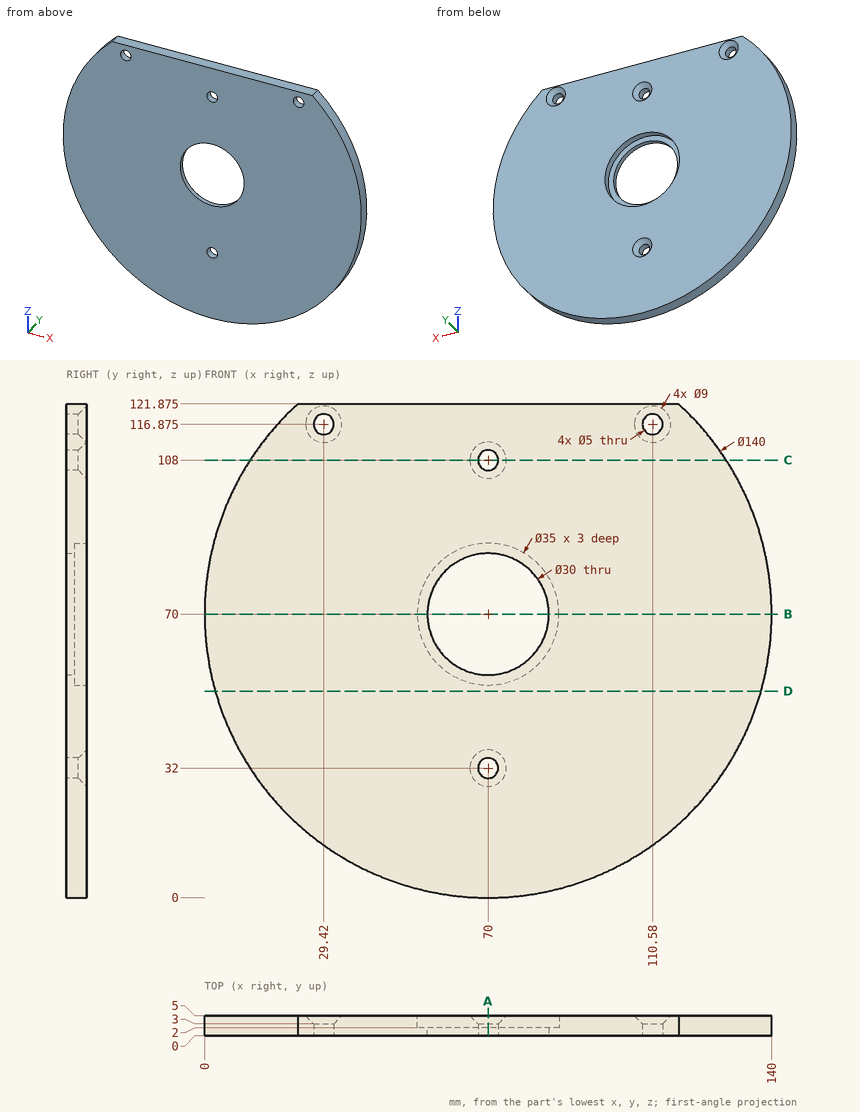
Geometry check sheet. Reference: drawing and pictorial views, mm from the part's lowest x, y, z. Round coordinates to 2 decimals unless told otherwise and drop trailing zeros. Write each loop counter-clockwise with the first axis right and the second up, starting at its lowest first coordinate (ties: lowest second). Pieces come first, ordered by that corner, then holes. Notation, with made-up numbers: (-12, -20) -> (10, -20) arc R19 ccw to (10, -6) -> close; hole circle Ø7 at (-25, 54). An arc over 180 degrees is marked (long way). Put each result on its own line as item: value.
1) Depth check by flat-ended pin: P1, Ø3, axis at y = 3.5, z = 49, coming from the -X side; P2, Ø6, axis at x = 29.42, z = 116.87, coming from the +Y side (1 decimal); P3, Ø3, axis at x = 70, z = 108, coming from the +Y side; P4, Ø6.5, axis at x = 70, z = 32, coming from the +Y side. Enter the tip coordinate at first touch or a pass-through.
Recorded:
P1: stops at x = 2.77
P2: stops at y = 3.5
P3: passes through
P4: stops at y = 3.75
2) Thickness scan on probe 1 along Z at (x, y) = (70, 0.8) (3 decimals); probe 2 along Z at (x, y) = (86.5, 0.7) (1 decimal); probe 3 along X at (y, z) = (0.3, 81.5). Record the ranges inside material, lowest first. Write a range as from..to.
Recorded:
probe 1: z = 0..29.5, 34.5..55, 85..105.5, 110.5..121.875
probe 2: z = 2..121.9
probe 3: x = 0.95..60.37, 79.63..139.05
3) Cross-section at C-C, the plane z = 108. Enter the section's corners in (x, y), plus the area to 3 significant figures.
Recorded:
outline: (11.21, 0) -> (67.5, 0) -> (67.5, 3) -> (65.5, 5) -> (11.21, 5) -> close; (72.5, 0) -> (128.79, 0) -> (128.79, 5) -> (74.5, 5) -> (72.5, 3) -> close
area: 559 mm2
4) Cross-section at D-D, the plane z = 51. Enter the section's corners in (x, y), plus the area to 3 significant figures.
Recorded:
outline: (2.63, 0) -> (137.37, 0) -> (137.37, 5) -> (2.63, 5) -> close
area: 674 mm2
5) Cross-section at B-B, the plane z = 70. Enter the section's corners in (x, y).
Recorded:
outline: (0, 0) -> (55, 0) -> (55, 2) -> (52.5, 2) -> (52.5, 5) -> (0, 5) -> close; (85, 0) -> (140, 0) -> (140, 5) -> (87.5, 5) -> (87.5, 2) -> (85, 2) -> close
6) Cross-section at A-A, the plane x = 70. Enter the section's corners in (y, z) (3 decimals), plus the area to 3 significant figures.
Recorded:
outline: (0, 0) -> (5, 0) -> (5, 27.5) -> (3, 29.5) -> (0, 29.5) -> close; (0, 34.5) -> (3, 34.5) -> (5, 36.5) -> (5, 52.5) -> (2, 52.5) -> (2, 55) -> (0, 55) -> close; (0, 85) -> (2, 85) -> (2, 87.5) -> (5, 87.5) -> (5, 103.5) -> (3, 105.5) -> (0, 105.5) -> close; (0, 110.5) -> (3, 110.5) -> (5, 112.5) -> (5, 121.875) -> (0, 121.875) -> close
area: 386 mm2
